from build123d import *

# Parameters (mm, degrees)
SKETCH1_W            = 25
SKETCH1_H            = 82
BOSS_EXTRUDE1_DEPTH  = 6
SKETCH2_W            = 45.31
SKETCH2_H            = 24
BOSS_EXTRUDE2_DEPTH  = 6
BOSS_EXTRUDE3_DEPTH  = 3
BOSS_EXTRUDE4_DEPTH  = 3
SKETCH5_W            = 41
SKETCH5_H            = 20
BOSS_EXTRUDE5_DEPTH  = 3
SKETCH6_W            = 48.1
SKETCH6_H            = 20
BOSS_EXTRUDE6_DEPTH  = 2.5
SKETCH7_W            = 41
SKETCH7_H            = 20
BOSS_EXTRUDE7_DEPTH  = 3
SKETCH8_W            = 48.1
SKETCH8_H            = 20
BOSS_EXTRUDE8_DEPTH  = 2.5
SKETCH9_R            = 1.5
CUT_EXTRUDE1_DEPTH   = 3
SKETCH10_R           = 1.5
CUT_EXTRUDE2_DEPTH   = 3
SKETCH11_W           = 46.1
SKETCH11_H           = 82
BOSS_EXTRUDE9_DEPTH  = 2
SKETCH12_R           = 3
BOSS_EXTRUDE10_DEPTH = 5
SKETCH13_R           = 1.4
BOSS_EXTRUDE11_DEPTH = 2.5
SKETCH14_W           = 2
SKETCH14_H           = 82
BOSS_EXTRUDE12_DEPTH = 42
SKETCH15_W           = 2.2
SKETCH15_H           = 82
BOSS_EXTRUDE13_DEPTH = 42
SKETCH16_W           = 20.8
SKETCH16_H           = 2
BOSS_EXTRUDE14_DEPTH = 42
SKETCH17_W           = 25
SKETCH17_H           = 82
BOSS_EXTRUDE15_DEPTH = 2


with BuildPart() as part:
    # Sketch1 → Boss-Extrude1 (new body)
    with BuildSketch(Plane(origin=(-72.6, 0, 0), x_dir=(0, 0, -1), z_dir=(1, 0, 0))):
        with Locations((40.5, 0)):
            Rectangle(SKETCH1_W, SKETCH1_H)
    extrude(amount=BOSS_EXTRUDE1_DEPTH)

    # Sketch2 → Boss-Extrude2 (add)
    with BuildSketch(Plane.XY.offset(-32.8)):
        with Locations((-95.245, 0)):
            Rectangle(SKETCH2_W, SKETCH2_H)
    extrude(amount=BOSS_EXTRUDE2_DEPTH)

    # Sketch3 → Boss-Extrude3 (add)
    with BuildSketch(Plane(origin=(0, 9, 0), x_dir=(1, 0, 0), z_dir=(0, 1, 0))):
        Polygon((-72.6, 32.8), (-72.6, 48.8), (-98.6, 32.8), align=None)
    extrude(amount=BOSS_EXTRUDE3_DEPTH)

    # Sketch4 → Boss-Extrude4 (add)
    with BuildSketch(Plane(origin=(0, -12, 0), x_dir=(1, 0, 0), z_dir=(0, 1, 0))):
        Polygon((-72.6, 32.8), (-72.6, 48.8), (-98.6, 32.8), align=None)
    extrude(amount=BOSS_EXTRUDE4_DEPTH)



with BuildPart() as body_2:
    # Sketch5 → Boss-Extrude5 (new body)
    with BuildSketch(Plane(origin=(-120.7, 0, 0), x_dir=(0, 0, -1), z_dir=(1, 0, 0))):
        with Locations((10.5, 28)):
            Rectangle(SKETCH5_W, SKETCH5_H)
    extrude(amount=BOSS_EXTRUDE5_DEPTH)


with BuildPart() as part_1:
    add(part.part)

    add(body_2.part)  # Boss-Extrude6 merges body 2
    # Sketch6 → Boss-Extrude6 (add)
    with BuildSketch(Plane.XY.offset(-31)):
        with Locations((-96.65, 28)):
            Rectangle(SKETCH6_W, SKETCH6_H)
    extrude(amount=BOSS_EXTRUDE6_DEPTH)



with BuildPart() as body_2_2:
    # Sketch7 → Boss-Extrude7 (new body)
    with BuildSketch(Plane(origin=(-120.7, 0, 0), x_dir=(0, 0, -1), z_dir=(1, 0, 0))):
        with Locations((10.5, -28)):
            Rectangle(SKETCH7_W, SKETCH7_H)
    extrude(amount=BOSS_EXTRUDE7_DEPTH)


with BuildPart() as part_2:
    add(part_1.part)

    add(body_2_2.part)  # Boss-Extrude8 merges body 2 2
    # Sketch8 → Boss-Extrude8 (add)
    with BuildSketch(Plane.XY.offset(-31)):
        with Locations((-96.65, -28)):
            Rectangle(SKETCH8_W, SKETCH8_H)
    extrude(amount=BOSS_EXTRUDE8_DEPTH)

    # Sketch9 → Cut-Extrude1 (cut)
    with BuildSketch(Plane(origin=(-117.7, 0, 0), x_dir=(0, 0, -1), z_dir=(1, 0, 0))):
        with Locations((-4, 24)):
            Circle(SKETCH9_R)
        with Locations((4, 24)):
            Circle(SKETCH9_R)
        with Locations((-4, 32)):
            Circle(SKETCH9_R)
        with Locations((4, 32)):
            Circle(SKETCH9_R)
        with Locations((-4, -32)):
            Circle(SKETCH9_R)
        with Locations((4, -32)):
            Circle(SKETCH9_R)
        with Locations((-4, -24)):
            Circle(SKETCH9_R)
        with Locations((4, -24)):
            Circle(SKETCH9_R)
    extrude(amount=-CUT_EXTRUDE1_DEPTH, mode=Mode.SUBTRACT)

    # Sketch10 → Cut-Extrude2 (cut)
    with BuildSketch(Plane.XY.offset(-26.8)):
        with Locations((-89.6, 4)):
            Circle(SKETCH10_R)
        with Locations((-89.6, -4)):
            Circle(SKETCH10_R)
        with Locations((-97.6, 4)):
            Circle(SKETCH10_R)
        with Locations((-97.6, -4)):
            Circle(SKETCH10_R)
    extrude(amount=-CUT_EXTRUDE2_DEPTH, mode=Mode.SUBTRACT)

    # Sketch11 → Boss-Extrude9 (add)
    with BuildSketch(Plane.XY.offset(-50.8)):
        with Locations((-95.65, 0)):
            Rectangle(SKETCH11_W, SKETCH11_H)
    extrude(amount=BOSS_EXTRUDE9_DEPTH)

    # Sketch12 → Boss-Extrude10 (add)
    with BuildSketch(Plane.XY.offset(-55.8)):
        with Locations((-115.15, -29)):
            Circle(SKETCH12_R)
        with Locations((-115.15, 29)):
            Circle(SKETCH12_R)
        with Locations((-76.15, -29)):
            Circle(SKETCH12_R)
        with Locations((-76.15, 29)):
            Circle(SKETCH12_R)
    extrude(amount=BOSS_EXTRUDE10_DEPTH)

    # Sketch13 → Boss-Extrude11 (add)
    with BuildSketch(Plane.XY.offset(-58.3)):
        with Locations((-115.15, -29)):
            Circle(SKETCH13_R)
        with Locations((-115.15, 29)):
            Circle(SKETCH13_R)
        with Locations((-76.15, -29)):
            Circle(SKETCH13_R)
        with Locations((-76.15, 29)):
            Circle(SKETCH13_R)
    extrude(amount=BOSS_EXTRUDE11_DEPTH)

    # Sketch14 → Boss-Extrude12 (add)
    with BuildSketch(Plane(origin=(-66.6, 0, 0), x_dir=(0, 0, -1), z_dir=(1, 0, 0))):
        with Locations((29, 0)):
            Rectangle(SKETCH14_W, SKETCH14_H)
    extrude(amount=BOSS_EXTRUDE12_DEPTH)

    # Sketch15 → Boss-Extrude13 (add)
    with BuildSketch(Plane(origin=(-66.6, 0, 0), x_dir=(0, 0, -1), z_dir=(1, 0, 0))):
        with Locations((51.9, 0)):
            Rectangle(SKETCH15_W, SKETCH15_H)
    extrude(amount=BOSS_EXTRUDE13_DEPTH)

    # Sketch16 → Boss-Extrude14 (add)
    with BuildSketch(Plane(origin=(-66.6, 0, 0), x_dir=(0, 0, -1), z_dir=(1, 0, 0))):
        with Locations((40.4, -40)):
            Rectangle(SKETCH16_W, SKETCH16_H)
    extrude(amount=BOSS_EXTRUDE14_DEPTH)

    # Sketch17 → Boss-Extrude15 (add)
    with BuildSketch(Plane(origin=(-24.6, 0, 0), x_dir=(0, 0, -1), z_dir=(1, 0, 0))):
        with Locations((40.5, 0)):
            Rectangle(SKETCH17_W, SKETCH17_H)
    extrude(amount=BOSS_EXTRUDE15_DEPTH)


solid = part_2.part
Verification items for the finished model (mm, model axes). A direction names the side the tool comes from. Give positions to 0.01 mm unless a question says otherwise; leave off trailing zeros. Loops run counter-clockwise (first coordinate to the right, second up) from the corner with the lowest first, then second, coordinate; pieces in that order, holes last. Notation, with made-up numbers: (37, -32.75) - (60, -32.75) arc R18 cw to (60, -14.75) - close; hole circle Ø2 at (1.25, 21.5). An arc over 180 degrees is marked (long way). Write item = value, one per line. Start each with the question number.
Q1. Depth check by flat-ended pin: P1, Ø6, axis at y = -33.5, z = -43.5, coming from the -X side; P2, Ø1.8, axis at x = -89.6, y = -4, coming from the -Z side; P3, Ø22, axis at y = -26, z = -14, coming from the +X side. Enter the tip coordinate at first touch or a pass-through.
Q2. Cross-section at A-A, the plane z = -4. Enter the section's corners in (x, y), and give its area (3 significant figures).
Q3. Mould release check, pull along Z, two halves, no side actions. Record for faces 4 (the face through (-119, -28, 10)), 5 (the face through (-72.6, 27, -38)), 6 (the face through (-115, -29, -58.3)): released by +Z, released by -Z, zero draft, split by the parting line, or undercut.
Q4. Tool access check on faces 1 (the face through (-107, -38, -29)), 2 (the face through (-98, 4, -29.8)), 3 (the face through (-74.815, -28.579, -57.067)). Record the directions out of +Z, -Z, +X, -X, +Y, -Y that give a thin tool (end or side, any length) a straight path to the whole face; none if there is none.
Q5. Thickness scan on line 1 (Y direction, x = -119.4, z = -4); line 2 (Z direction, x = -111, y = 2); line 3 (Z direction, x = -65, y = 22). Record the ranges inside material, lowest first.
Q6. Cross-section at B-B, the plane y = 14. Enter the section's corners in (x, z), and give its area (3 significant figures).
Q7. Cross-section at D-D, the plane x = -46.5. Enter the section's corners in (y, z).
Q8. Cross-section at C-C, the plane x = -84. Enter the section's corners in (y, z), and give its area (3 significant figures).
Answer key:
q1.P1 = -72.6
q1.P2 = -50.8
q1.P3 = -117.7
q2.outline = (-120.7, -38) - (-117.7, -38) - (-117.7, -33.5) - (-120.7, -33.5) - close; (-120.7, -30.5) - (-117.7, -30.5) - (-117.7, -25.5) - (-120.7, -25.5) - close; (-120.7, -22.5) - (-117.7, -22.5) - (-117.7, -18) - (-120.7, -18) - close; (-120.7, 18) - (-117.7, 18) - (-117.7, 22.5) - (-120.7, 22.5) - close; (-120.7, 25.5) - (-117.7, 25.5) - (-117.7, 30.5) - (-120.7, 30.5) - close; (-120.7, 33.5) - (-117.7, 33.5) - (-117.7, 38) - (-120.7, 38) - close
q2.area = 84.0 mm^2
q3.face_4 = released by +Z
q3.face_5 = undercut
q3.face_6 = released by -Z
q4.face_1 = +Z, -X, -Y
q4.face_2 = +Z
q4.face_3 = -Z
q5.line_1 = -38 to -33.5, -30.5 to -25.5, -22.5 to -18, 18 to 22.5, 25.5 to 30.5, 33.5 to 38
q5.line_2 = -50.8 to -48.8, -32.8 to -26.8
q5.line_3 = -53 to -50.8, -30 to -28
q6.outline = (-118.7, -50.8) - (-72.6, -50.8) - (-72.6, -53) - (-22.6, -53) - (-22.6, -28) - (-72.6, -28) - (-72.6, -48.8) - (-118.7, -48.8) - close; hole (-66.6, -50.8) - (-24.6, -50.8) - (-24.6, -30) - (-66.6, -30) - close
q6.area = 469 mm^2
q7.outline = (-41, -53) - (41, -53) - (41, -50.8) - (-39, -50.8) - (-39, -30) - (41, -30) - (41, -28) - (-41, -28) - close
q8.outline = (-41, -50.8) - (41, -50.8) - (41, -48.8) - (-41, -48.8) - close; (-38, -31) - (-18, -31) - (-18, -28.5) - (-38, -28.5) - close; (-12, -41.78) - (-9, -41.78) - (-9, -32.8) - (9, -32.8) - (9, -41.78) - (12, -41.78) - (12, -26.8) - (-12, -26.8) - close; (18, -31) - (38, -31) - (38, -28.5) - (18, -28.5) - close
q8.area = 462 mm^2
